Can you work these out from the model? Positions are in its coordinate system, mm. Round coordinates to 2 decimals unless told otherwise and drop trailing zeros. Write each loop counter-clockwise with the first axis right and the second up, starting at its lowest first coordinate (ties: lowest second). Pieces come first, ordered by that corner, then holes. Notation, with made-up numbers: M -27.75,30.5 L 20.25,30.5 A23 ccw 20.25,52.5 Z; hole C 74.25,-9 d8. An arc over 180 degrees is marked long. Answer in a Markdown table with one row per item. Add a question column.
(1) If we mould it in two halves opening along Z, with no side actions, what happens to faces 1 (the face through (172, 0, -12)), 2 (the face through (258.549, 0.986, -10.654))? For each: released by +Z, released by -Z, zero draft, split by the parting line, or undercut.
(2) If I drill on probe 1 along Z at (x, y) = (290, 0.65); probe 2 along Z at (x, y) = (90, 1.35); probe 3 along Z at (x, y) = (315, 0.7), over which ranges is the centre line in solid material (lowest first)?
(3) Suppose I cut it at B-B, the plane y = 1.35. Count the separate pieces of the cut face and the enclosed holes in it, then the cut area to 3 significant figures.
(4) Suppose I cut it at A-A, the plane x = 120. Write out the boundary of the cut face in (y, z).
(5) I'm going to push a flat-ended pin straight in: pin 1 (4 mm diameter, centred on x = 330, z = -21.25, fed in from +Y). Where does the tip first touch, or does it pass through?
Autodesk Inventor part; units mm, degrees
ref_plane "YZ Plane" through (0, 0, 0) normal (1, 0, 0) x (0, 1, 0)
ref_plane "XZ Plane" through (0, 0, 0) normal (0, 1, 0) x (-1, 0, 0)
ref_plane "XY Plane" through (0, 0, 0) normal (0, 0, 1) x (1, 0, 0)
sketch "スケッチ1" plane through (0, 0, 0) normal (0, 1, 0) x (-1, 0, 0)
  line L0 (0, 0) -> (-340, 0)
  line L1 (-340, 0) -> (-340, -25)
  line L2 (-340, -25) -> (0, -25)
  line L3 (0, -25) -> (0, 0)
  dimension "d0" = 340
  dimension "d1" = 25
extrude "押し出し1" add sketch "スケッチ1" along normal blind 2
sketch "スケッチ2" plane through (0, 2, 0) normal (0, 1, 0) x (1, 0, 0)
  line L0 (0, 25) -> (0, 0)
  line L1 (0, 12.5) -> (340, 12.5)
  line L2 (340, 0) -> (340, 25)
  line L3 (0, 12.5) -> (340, 12.5)
  line L4 (340, 12.5) -> (340, 17.5)
  line L5 (340, 17.5) -> (0, 17.5)
  line L6 (0, 17.5) -> (0, 12.5)
  line L7 (0, 0) -> (0, 25)
  line L8 (340, 25) -> (340, 0)
  line L9 (340, 7.5) -> (0, 7.5)
  line L10 (0, 0) -> (340, 0)
  line L11 (340, 0) -> (340, 25)
  line L12 (340, 25) -> (0, 25)
  line L13 (0, 25) -> (0, 0)
  point P0 (0, 17.5)
  point P1 (0, 7.5)
  dimension "d4" = 5
extrude "押し出し2" cut sketch "スケッチ2" against normal blind 1 contours L12 L2 L5 L0 | L9 L2 L10 L0
sketch "スケッチ3" plane through (0, 1, 0) normal (0, 1, 0) x (1, 0, 0)
  line L0 (0, 0) -> (0, 7.5)
  line L1 (0, 3.75) -> (340, 3.75)
  line L2 (340, 7.5) -> (340, 0)
  line L3 (340, 7.5) -> (340, 17.5)
  line L4 (340, 12.5) -> (0, 12.5)
  line L5 (0, 17.5) -> (0, 7.5)
  point P0 (10, 3.75)
  point P1 (80, 3.75)
  point P2 (150, 3.75)
  point P3 (220, 3.75)
  point P4 (290, 3.75)
  point P5 (10, 21.25)
  point P6 (80, 21.25)
  point P7 (150, 21.25)
  point P8 (220, 21.25)
  point P9 (290, 21.25)
  point P10 (330, 3.75)
  point P11 (330, 21.25)
  dimension "d7" = 10
  dimension "d8" = 70
  dimension "d11" = 70
  dimension "d38" = 10
hole "穴1" at (10, 1, -3.75) at (80, 1, -3.75) at (150, 1, -3.75) at (220, 1, -3.75) at (290, 1, -3.75) at (10, 1, -21.25) at (80, 1, -21.25) at (150, 1, -21.25) at (220, 1, -21.25) at (290, 1, -21.25) at (330, 1, -21.25) at (330, 1, -3.75) direction (0, -1, 0) diameter 3.1 end through all
sketch "スケッチ4" plane through (0, 2, 0) normal (0, 1, 0) x (1, 0, 0)
  line L0 (340, 0) -> (340, 25)
  line L1 (340, 12.5) -> (0, 12.5)
  line L2 (0, 17.5) -> (0, 7.5)
  point P0 (0, 0)
  point P1 (330, 12.5)
  point P2 (315, 12.5)
  point P3 (300, 12.5)
  point P4 (285, 12.5)
  point P5 (270, 12.5)
  point P6 (255, 12.5)
  point P7 (240, 12.5)
  point P8 (225, 12.5)
  point P9 (210, 12.5)
  point P10 (195, 12.5)
  point P11 (180, 12.5)
  point P12 (165, 12.5)
  point P13 (150, 12.5)
  point P14 (135, 12.5)
  point P15 (120, 12.5)
  point P16 (105, 12.5)
  point P17 (90, 12.5)
  point P18 (75, 12.5)
  point P19 (60, 12.5)
  point P20 (45, 12.5)
  point P21 (30, 12.5)
  point P22 (15, 12.5)
  point P23 (0, 12.5)
  dimension "d23" = 10
  dimension "d26" = 15
hole "穴2" at (330, 2, -12.5) at (315, 2, -12.5) at (300, 2, -12.5) at (285, 2, -12.5) at (270, 2, -12.5) at (255, 2, -12.5) at (240, 2, -12.5) at (225, 2, -12.5) at (210, 2, -12.5) at (195, 2, -12.5) at (180, 2, -12.5) at (165, 2, -12.5) at (150, 2, -12.5) at (135, 2, -12.5) at (120, 2, -12.5) at (105, 2, -12.5) at (90, 2, -12.5) at (75, 2, -12.5) at (60, 2, -12.5) at (45, 2, -12.5) at (30, 2, -12.5) at (15, 2, -12.5) at (0, 2, -12.5) direction (0, -1, 0) diameter 8 depth 8 tip angle 118
equation "\"d0\" = polygon_len1"
equation "\"d4\" = 0.5 * polygon_wid3"
properties part number "link1plate2" material "アルミニウム 6061"
Calculated:
| question | item | result |
|---|---|---|
| 1 | face 1 | zero draft |
| 1 | face 2 | undercut |
| 2 | probe 1 | -25 to -22.8, -19.7 to -5.3, -2.2 to 0 |
| 2 | probe 2 | -17.5 to -16.5, -8.5 to -7.5 |
| 2 | probe 3 | -25 to -16.5, -8.5 to 0 |
| 3 | separate pieces | 1 |
| 3 | enclosed holes | 22 |
| 3 | area | 2,270 mm² |
| 4 | outline | M 0,-25 L 1,-25 L 1,-17.5 L 2,-17.5 L 2,-16.5 L 0,-16.5 Z; M 0,-8.5 L 2,-8.5 L 2,-7.5 L 1,-7.5 L 1,0 L 0,0 Z |
| 5 | pin 1 | y = 1 |
